The figure shows three views and two pictorial views of one solid part (mm, origin at its lowest corner). Answer the questions. A direction names the side the tool comes from. Coordinates: 2 decimals unless noted, no trailing zeros. Write each loop counter-clockwise with the first axis right and the second up, starting at its lowest first coordinate (ties: lowest second). Pieces come first, ordered by that corner, then holes.
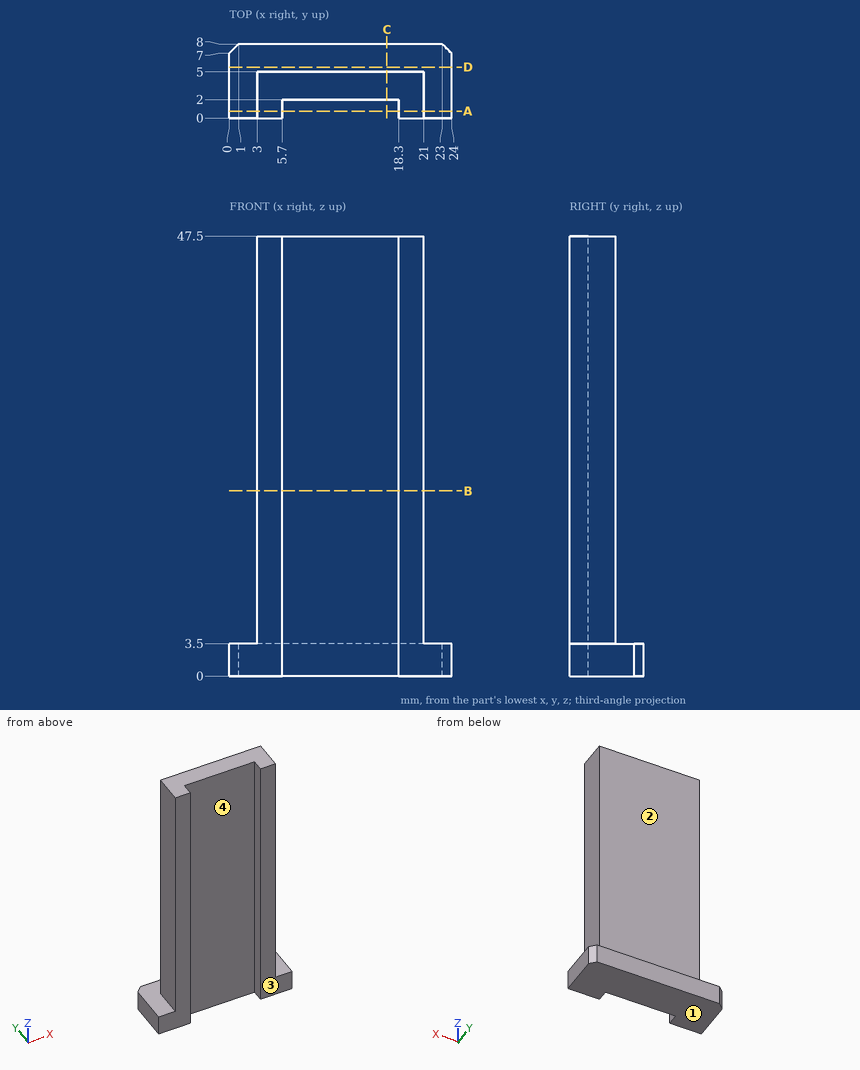
1. Section A-A on y = 0.75 is taken. Give the vertices of the cut face in (x, z).
Results found:
outline: (0, 0) - (5.7, 0) - (5.7, 47.5) - (3, 47.5) - (3, 3.5) - (0, 3.5) - close; (18.3, 0) - (24, 0) - (24, 3.5) - (21, 3.5) - (21, 47.5) - (18.3, 47.5) - close
2. Flat-ended cylindrical pins translate along their axes: P1, Ø2, axis at y = 0.5, z = 17, coming from the +X side; P2, Ø3, axis at x = 15.5, z = 28, coming from the -Y side; P3, Ø5, axis at x = 9, z = 20.5, coming from the +Y side. Find the tip coordinate at first contact, or state that the pin passes through.
Results found:
P1: stops at x = 21
P2: stops at y = 2
P3: stops at y = 5
3. Section D-D on y = 5.5 is taken. Give the vertices of the cut face in (x, z), then the cut area to 3 significant figures.
Results found:
outline: (0, 0) - (24, 0) - (24, 3.5) - (0, 3.5) - close
area: 84.0 mm2
4. Section B-B on z = 20 is taken. Give the vertices of the cut face in (x, y).
Results found:
outline: (3, 0) - (5.7, 0) - (5.7, 2) - (18.3, 2) - (18.3, 0) - (21, 0) - (21, 5) - (3, 5) - close
5. Section C-C on x = 17 is taken. Give the vertices of the cut face in (y, z), then the cut area to 3 significant figures.
Results found:
outline: (2, 0) - (8, 0) - (8, 3.5) - (5, 3.5) - (5, 47.5) - (2, 47.5) - close
area: 153 mm2
6. A tool of negligible diameter and unlimited length cuts with its end or side. For the marked faces 1 and 2, from which of +Z, -Z, +X, -X, +Y, -Y can it reach the whole face along a straight path? Write none if from no direction.
Results found:
face 1: -Z, +X, -X, +Y, -Y
face 2: +Z, +X, -X, +Y
7. Find the intervals of material crossed by L1, parallel to X at y = 0.5, z = 3; L2, parallel to X at y = 0.5, z = 19; L3, parallel to Z at x = 2.25, y = 1.25, in increasing order.
Results found:
L1: x = 0 to 5.7, 18.3 to 24
L2: x = 3 to 5.7, 18.3 to 21
L3: z = 0 to 3.5
8. For a pull along X with two mould halves and no side action, classify the marked faces 3 and 4 as pulls with the +X half, pulls with the -X half, needs draft (parallel to the pull), parting line crosses it, or undercut.
Results found:
face 3: needs draft
face 4: undercut
